from build123d import *

# Parameters (mm, degrees)
SKETCH1_W            = 280
SKETCH1_H            = 75
BOSS_EXTRUDE1_DEPTH  = 15
SKETCH8_R            = 5
CUT_EXTRUDE4_DEPTH   = 146.709471209
SKETCH10_R           = 5
CUT_EXTRUDE6_DEPTH   = 146.709471209
SKETCH9_W            = 165
SKETCH9_H            = 65
CUT_EXTRUDE5_DEPTH   = 4
SHELL2_OUTLINE_W     = 277
SHELL2_OUTLINE_H     = 69
SHELL2_OUTLINE_R     = 5
SHELL2_DEPTH         = 8
SHELL2_START         = 8
SHELL2_2_OUTLINE_W   = 17
SHELL2_2_OUTLINE_H   = 69
SHELL2_2_OUTLINE_W_2 = 89
SHELL2_2_OUTLINE_R   = 5
SHELL2_2_DEPTH       = 4
SKETCH11_W           = 5
SKETCH11_H           = 5
BOSS_EXTRUDE4_DEPTH  = 2
FILLET1_R            = 1


# Read off the part's stored shape, not the designer's step: Shell2
with BuildPart() as part:
    # Sketch1 → Boss-Extrude1 (new body)
    with BuildSketch(Plane(origin=(0, 0, 0), x_dir=(1, 0, 0), z_dir=(0, 1, 0))):
        Rectangle(SKETCH1_W, SKETCH1_H)
    extrude(amount=BOSS_EXTRUDE1_DEPTH)

    # Sketch8 → Cut-Extrude4 (cut, through all)
    with BuildSketch(Plane(origin=(0, 15, 0), x_dir=(1, 0, 0), z_dir=(0, 1, 0))):
        with Locations(Location((121.166163263, 0, 0), (0, 0, 270))):
            Circle(SKETCH8_R)
    extrude(amount=-CUT_EXTRUDE4_DEPTH, mode=Mode.SUBTRACT)

    # Sketch10 → Cut-Extrude6 (cut, through all)
    with BuildSketch(Plane(origin=(0, 15, 0), x_dir=(1, 0, 0), z_dir=(0, 1, 0))):
        with Locations(Location((26.698268473, 0, 0), (0, 0, 270))):
            Circle(SKETCH10_R)
    extrude(amount=-CUT_EXTRUDE6_DEPTH, mode=Mode.SUBTRACT)

    # Sketch9 → Cut-Extrude5 (cut)
    with BuildSketch(Plane(origin=(0, 15, 0), x_dir=(1, 0, 0), z_dir=(0, 1, 0))):
        with Locations((-37.5, 0)):
            Rectangle(SKETCH9_W, SKETCH9_H)
    extrude(amount=-CUT_EXTRUDE5_DEPTH, mode=Mode.SUBTRACT)

    # Shell2 outline → Shell2 (cut)
    with BuildSketch(Plane(origin=(0, 0, 0), x_dir=(1, 0, 0), z_dir=(0, 1, 0))):
        with Locations((-1.5, 0)):
            Rectangle(SHELL2_OUTLINE_W, SHELL2_OUTLINE_H)
        with Locations((26.698268473, 0)):
            Circle(SHELL2_OUTLINE_R, mode=Mode.SUBTRACT)
        with Locations((121.166163263, 0)):
            Circle(SHELL2_OUTLINE_R, mode=Mode.SUBTRACT)
    extrude(amount=SHELL2_DEPTH, mode=Mode.SUBTRACT)

    # Shell2 2 outline → Shell2 2 (cut)
    # profile 1 of 2: a face of its own
    with BuildSketch(Plane(origin=(0, 0, 0), x_dir=(1, 0, 0), z_dir=(0, 1, 0)).offset(SHELL2_START)):
        with Locations((-131.5, 0)):
            Rectangle(SHELL2_2_OUTLINE_W, SHELL2_2_OUTLINE_H)
    # profile 2 of 2: a face of its own
    with BuildSketch(Plane(origin=(0, 0, 0), x_dir=(1, 0, 0), z_dir=(0, 1, 0)).offset(SHELL2_START)):
        with Locations((92.5, 0)):
            Rectangle(SHELL2_2_OUTLINE_W_2, SHELL2_2_OUTLINE_H)
        with Locations((121.166163263, 0)):
            Circle(SHELL2_2_OUTLINE_R, mode=Mode.SUBTRACT)
    extrude(amount=SHELL2_2_DEPTH, mode=Mode.SUBTRACT)

    # Sketch11 → Boss-Extrude4 (add)
    with BuildSketch(Plane.XY.offset(37.5)):
        with Locations((80, 7.5)):
            Rectangle(SKETCH11_W, SKETCH11_H)
        with Locations((125.124035555, 7.5)):
            Rectangle(SKETCH11_W, SKETCH11_H)
    extrude(amount=BOSS_EXTRUDE4_DEPTH)

    # Fillet1
    fillet1_edges = [part.edges().sort_by_distance(p)[0] for p in [
        (82.5, 7.5, 39.5),
        (80, 10, 39.5),
        (77.5, 7.5, 39.5),
        (80, 5, 39.5),
        (127.624035555, 7.5, 39.5),
        (125.124035555, 10, 39.5),
        (122.624035555, 7.5, 39.5),
        (125.124035555, 5, 39.5),
    ]]
    fillet(fillet1_edges, radius=FILLET1_R)


solid = part.part
Design review of the part built by this model. Coordinates are the model's own, in mm. A direction names the side the tool comes from. Coordinates: 2 decimals unless noted, no trailing zeros. Order: outer loops, then holes, each group sorted by start corner. A loop starts at its lowest first (then second) coordinate and runs counter-clockwise, first axis right, second up. Notation, with made-up numbers: (20.5, -39.5) -> (27.5, -39.5) arc R27 cw to (27.5, -12.5) -> close; hole circle Ø10 at (44, 49.5). An arc over 180 degrees is marked (long way). Use one line per item in the form item = value. Start each with the question number.
(1) The part is to be moulded in two halves that separate along Z. For faces 1 (the flat face through (-132, 12, 0)), 2 (the flat face through (140, 7, 1)), 3 (the flat face through (-2, 7, -37.5)), say which applies: +Z half, -Z half, draft (parallel to the pull), parting line (faces both ways), or undercut.
(2) For faces 4 (the flat face through (-3, 5, 34.5)), 5 (the flat face through (-39, 8, 0)), 6 (the flat face through (-39, 11, 0)), list the 3-axis set-ups (+Z, -Z, +X, -X, +Y, -Y) from which the entire face can be reached by the end or side of a thin tool; tool diameter is ignored.
(3) Insertion check: pin 1 (0.5 mm diameter, centred on x = 81, z = 38, fed in from -Y); pin 2 (0.5 mm diameter, centred on y = 7.5, z = 38, fed in from +X); pin 3 (1.1 mm diameter, centred on x = 124.5, z = 38, fed in from +Y); pin 4 (8 mm diameter, centred on x = -19, z = -26, fed in from -Y). Each pin has a flat end and moves straight along its axis. Give the tip position at first contact, or say it passes through.
(4) Add section D-D on z = -21. State the section outline as (x, y) points, plus the area to 3 significant figures.
(5) Add section C-C on y = 2.5. State the section outline as (x, z) points.
(6) For probe 1 along X at (y, z) = (10.3, 0); probe 2 along X at (y, z) = (14.35, 0); probe 3 along Z at (x, y) = (-30.5, 5.5), list the stretches that pass through material, from the lowest coordinate up.
(7) Add section B-B on x = 12. State the section outline as (y, z) points, plus the area to 3 significant figures.
(8) Add section A-A on z = 0. State the section outline as (x, y) points, plus the area to 3 significant figures.
Answer block:
q1.face_1 = undercut
q1.face_2 = draft
q1.face_3 = -Z half
q2.face_4 = -Y
q2.face_5 = -X, -Y
q2.face_6 = +Y
q3.pin_1 = 5
q3.pin_2 = 127.62
q3.pin_3 = 15
q3.pin_4 = 8
q4.outline = (-140, 12) -> (-123, 12) -> (-123, 8) -> (48, 8) -> (48, 12) -> (137, 12) -> (137, 0) -> (140, 0) -> (140, 15) -> (45, 15) -> (45, 11) -> (-120, 11) -> (-120, 15) -> (-140, 15) -> close
q4.area = 900 mm²
q5.outline = (-140, -37.5) -> (140, -37.5) -> (140, 37.5) -> (-140, 37.5) -> (-140, 34.5) -> (137, 34.5) -> (137, -34.5) -> (-140, -34.5) -> close
q6.probe_1 = -123 to 21.7, 31.7 to 48, 137 to 140
q6.probe_2 = -140 to -120, 45 to 116.17, 126.17 to 140
q6.probe_3 = -37.5 to -34.5, 34.5 to 37.5
q7.outline = (0, -37.5) -> (15, -37.5) -> (15, -32.5) -> (11, -32.5) -> (11, 32.5) -> (15, 32.5) -> (15, 37.5) -> (0, 37.5) -> (0, 34.5) -> (8, 34.5) -> (8, -34.5) -> (0, -34.5) -> close
q7.area = 313 mm²
q8.outline = (-140, 12) -> (-123, 12) -> (-123, 8) -> (21.7, 8) -> (21.7, 11) -> (-120, 11) -> (-120, 15) -> (-140, 15) -> close; (31.7, 8) -> (48, 8) -> (48, 12) -> (116.17, 12) -> (116.17, 15) -> (45, 15) -> (45, 11) -> (31.7, 11) -> close; (126.17, 12) -> (137, 12) -> (137, 0) -> (140, 0) -> (140, 15) -> (126.17, 15) -> close
q8.area = 840 mm²
